Verification items for the finished model (mm, model axes). A direction names the side the tool comes from. Round coordinates to 2 decimals unless told otherwise and drop trailing zeros. Order: outer loops, then holes, each group sorted by start corner. A loop starts at its lowest first (then second) coordinate and runs counter-clockwise, first axis right, second up. Notation, with made-up numbers: (-31, -36) -> (8, -36) arc R33 ccw to (8, -8) -> close; hole circle Ø7 at (33, -14). An arc over 180 degrees is marked (long way). Put each result on its own line as item: value.
```python
from build123d import *

# Parameters (mm, degrees)
REVOLUTION_ANGLE = 100
FILLET_R         = 8
PAD_DEPTH        = 8
POCKET_DEPTH     = 2
CHAMFER_SIZE     = 1
SKETCH005_W      = 3
SKETCH005_H      = 7
POCKET001_DEPTH  = 81.8615815525
POCKET002_DEPTH  = 78.501
FILLET001_R      = 3
FILLET002_R      = 1


with BuildPart() as part:
    # Sketch → Revolution (revolve, symmetric)
    with BuildSketch(Plane.XY) as revolution_sk:
        with BuildLine():
            ThreePointArc((27.5, 224.008535095), (0, 250), (-27.5, 224.008535095))
            Line((-34.5, 100), (-27.5, 224.008535095))
            Line((-34.5, 100), (-32.5, 100))
            Line((-32.5, 100), (-25.0114058168, 223.77))
            ThreePointArc((25.0114058168, 223.77), (0, 247.3138512729), (-25.0114058168, 223.77))
            Line((25.0114058168, 223.77), (32.5, 100))
            Line((32.5, 100), (34.5, 100))
            Line((34.5, 100), (27.5, 224.008535095))
        make_face()
    revolve(axis=Axis((0, 0, 0), (1, 0, 0)), revolution_arc=REVOLUTION_ANGLE / 2)
    revolve(revolution_sk.sketch, axis=Axis((0, 0, 0), (-1, 0, 0)), revolution_arc=REVOLUTION_ANGLE / 2)

    # Fillet
    fillet_edges = [part.edges().sort_by_distance(p)[0] for p in [
        (33.5, 64.278761, 76.604444),
        (-33.5, 64.278761, 76.604444),
    ]]
    fillet(fillet_edges, radius=FILLET_R)

    # Sketch002 (on Face5 of Fillet) → Pad (new body)
    with BuildSketch(Plane(origin=(0, 0, 0), x_dir=(1, 0, 0), z_dir=(0, -0.7660444431, 0.6427876097))):
        Polygon((-43.3941714588, 132.6975053664), (-46.5, 121.1063954509), (-33.2488189206, 107.8552143715), (-31, 145.091676825), align=None)
        Polygon((43.3941714588, 132.6975053664), (46.5, 121.1063954509), (33.2488189206, 107.8552143715), (31, 145.091676825), align=None)
        Polygon((28, 194.1063954509), (32, 198.1063954509), (32, 206.1063954509), (28, 210.1063954509), (24, 206.1063954509), (24, 198.1063954509), align=None)
        Polygon((-28, 194.1063954509), (-24, 198.1063954509), (-24, 206.1063954509), (-28, 210.1063954509), (-32, 206.1063954509), (-32, 198.1063954509), align=None)
    extrude(amount=-PAD_DEPTH)

    # Sketch003 (on Face47 of Pad) → Pocket (cut)
    with BuildSketch(Plane(origin=(0, 0, 0), x_dir=(1, 0, 0), z_dir=(0, -0.7660444431, 0.6427876097))):
        Polygon((35, 146.8697948557), (45, 97.88), (47.9393876913, 98.48), (37.9393876913, 147.4697948557), align=None)
        Polygon((-47.9393876913, 98.4800000001), (-45, 97.88), (-35, 146.8697948557), (-37.9393876913, 147.4697948558), align=None)
    extrude(amount=-POCKET_DEPTH, mode=Mode.SUBTRACT)

    # Chamfer
    chamfer_edges = [part.edges().sort_by_distance(p)[0] for p in [
        (42.094426, 81.707526, 97.375238),
        (38.89944, 82.126736, 97.874832),
        (-38.89944, 82.126736, 97.874832),
        (-42.094426, 81.707526, 97.375238),
    ]]
    chamfer(chamfer_edges, length=CHAMFER_SIZE)

    # Sketch005 (on Face6 of Chamfer) → Pocket001 (cut, through all)
    with BuildSketch(Plane(origin=(0, 6.128355545, -5.1423008775), x_dir=(-1, 0, 0), z_dir=(0, 0.7660444431, -0.6427876097))):
        with Locations((-36.0477122259, 125.0785244639)):
            Rectangle(SKETCH005_W, SKETCH005_H)
        with Locations((36.0477122259, 125.0785244639)):
            Rectangle(SKETCH005_W, SKETCH005_H)
    extrude(amount=-POCKET001_DEPTH, mode=Mode.SUBTRACT)

    # Sketch006 (on Face54 of Pocket001) → Pocket002 (cut, through all)
    with BuildSketch(Plane(origin=(-32, 0, 0), x_dir=(0, -1, 0), z_dir=(-1, 0, 0))):
        Polygon((-140.4082247347, 149.7281591854), (-136.6575524936, 145.0449489894), (-134.3159473956, 146.92028511), (-138.0666196367, 151.6034953059), align=None)
    extrude(amount=-POCKET002_DEPTH, mode=Mode.SUBTRACT)

    # Fillet001
    fillet001_edges = [part.edges().sort_by_distance(p)[0] for p in [
        (46.5, 80.909868, 90.201731),
        (43.394171, 88.36049, 99.081036),
        (-43.394171, 88.36049, 99.081036),
        (-46.5, 80.909868, 90.201731),
    ]]
    fillet(fillet001_edges, radius=FILLET001_R)

    # Fillet002
    fillet002_edges = [part.edges().sort_by_distance(p)[0] for p in [
        (32, 135.546815, 155.315508),
        (32, 130.404514, 149.187153),
        (-32, 130.404514, 149.187153),
        (-32, 135.546815, 155.315508),
    ]]
    fillet(fillet002_edges, radius=FILLET002_R)


solid = part.part
```
Item 1: Sectioned sample at B-B, the plane x = -12.5. Record the boundary of the cut face in (y, z).
Geometry check:
outline: (156.82, -186.89) -> (158.77, -189.21) arc R247 ccw to (158.77, 189.21) -> (156.82, 186.89) arc R243.97 cw to start
Item 2: Tool access check on faces 1 (the face through (-42.55, 82.24, 97.22)), 2 (the face through (27.95, 119.855, -142.837)), 3 (the face through (34.548, 83, 93)), 4 (the face through (-24, 133, 152)), 5 (the face through (32, 133, 152)). Record the directions out of +Z, -Z, +X, -X, +Y, -Y that give a thin tool (end or side, any length) a straight path to the whole face; none if there is none.
Geometry check:
face 1: +Z, -Y
face 2: -Z, +X, -X, -Y
face 3: none
face 4: +Z, -Z, -Y
face 5: +Z, +X, +Y, -Y
Item 3: Release check for a two-part mould opening along Z. For faces 6 (the face through (39.175, 87.503, 91.837)), 7 (the face through (24, 133, 152)), 8 (the face through (44.062, 81.229, 96.806)) record: pulls with the +Z half, pulls with the -Z half, needs draft (parallel to the pull), parting line crosses it, or undercut.
Geometry check:
face 6: undercut
face 7: needs draft
face 8: pulls with the +Z half
Item 4: Sectioned sample at A-A, the plane x = 6.5. Record the boundary of the cut face in (y, z).
Geometry check:
outline: (158.42, -188.8) -> (160.2, -190.92) arc R249.22 ccw to (160.2, 190.92) -> (158.42, 188.8) arc R246.46 cw to start
Item 5: Material ranges on line 1 along X through (y, z) = (99, -15); line 2 along X through (y, z) = (118.5, 6); line 3 along Z through (x, y) = (14.5, 166), recorded low to high.
Geometry check:
line 1: -34.49 to -32.49, 32.49 to 34.49
line 2: -33.45 to -31.37, 31.37 to 33.45
line 3: -181.38 to -177.04, 177.04 to 181.38
Item 6: Depth check by flat-ended pin: pin 1 Ø9 at (y, z) = (132, 150.5) entering from -X; pin 2 Ø12.5 at (y, z) = (132.5, 154) entering from +X; pin 3 Ø5.5 at (y, z) = (83.5, 95) entering from +X; pin 4 Ø10 at (y, z) = (223.5, -130) entering from -X. Enter the tip coordinate at first touch or a pass-through.
Geometry check:
pin 1: x = -32
pin 2: x = 32
pin 3: x = 45.81
pin 4: through
